Source: three-view drawing plus pictorial views. Frame: mm from the lowest corner of the part. Give positions to 0.01 mm unless a question says otherwise; leave off trailing zeros. Order: outer loops, then holes, each group sorted by start corner. A loop starts at its lowest first (then second) coordinate and runs counter-clockwise, first axis right, second up. Notation, with made-up numbers: (34, 32) -> (80, 32) arc R6 ccw to (80, 38) -> close; hole circle Ø6 at (32, 46). An arc over 180 degrees is marked (long way). Answer in a Markdown table with one row per item. Add a question column.
Q1. Line query: line 1 along X through (y, z) = (30, 3.35) (1 decimal); line 2 along X through (y, z) = (80, 0.5) (1 decimal); line 3 along X through (y, z) = (75.5, 0.9) (1 decimal). Output: solid intervals per line, ascending. Write a range as from..to.
Q2. Cut plane C-C on y = 56. Return the cut outline in (x, z).
Q3. Cut plane D-D on x = 119. Return the cut outline in (y, z).
Q4. Contact query for flat-ended pins moving along their axis: P1, Ø2.5, axis at y = 1.5, z = 1.5, coming from the -X side; P2, Ø2.5, axis at y = 89, z = 2.5, coming from the -X side (1 decimal); P3, Ø2.5, axis at y = 1.5, z = 1.5, coming from the +X side. Output: stop coordinate, or through.
Q5. Cut plane A-A on y = 11. Return the cut outline in (x, z) (1 decimal).
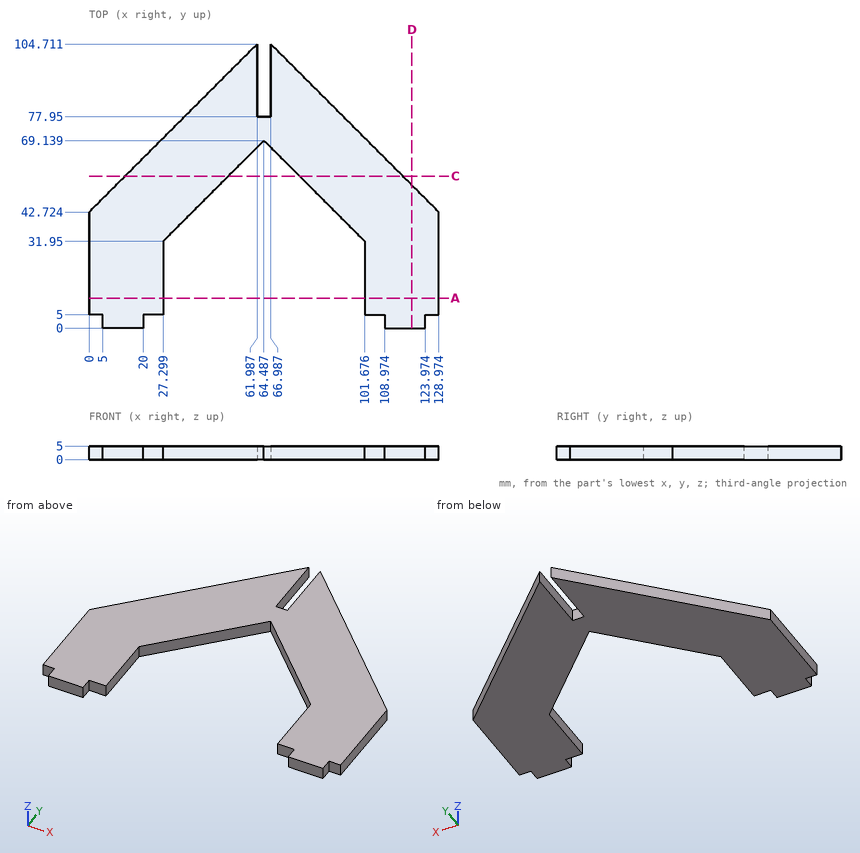
Completed:
| question | item | result |
|---|---|---|
| 1 | line 1 | x = 0..27.3, 101.7..129 |
| 1 | line 2 | x = 37.3..62, 67..91.7 |
| 1 | line 3 | x = 32.8..96.2 |
| 2 | outline | (13.28, 0) -> (51.35, 0) -> (51.35, 5) -> (13.28, 5) -> close; (77.63, 0) -> (115.7, 0) -> (115.7, 5) -> (77.63, 5) -> close |
| 3 | outline | (0, 0) -> (52.7, 0) -> (52.7, 5) -> (0, 5) -> close |
| 4 | P1 | stops at x = 5 |
| 4 | P2 | stops at x = 45 |
| 4 | P3 | stops at x = 123.97 |
| 5 | outline | (0, 0) -> (27.3, 0) -> (27.3, 5) -> (0, 5) -> close; (101.7, 0) -> (129, 0) -> (129, 5) -> (101.7, 5) -> close |
